Model file for the job. Use its own axes, mm. A direction names the side the tool comes from. Coordinates: 2 decimals unless noted, no trailing zeros. Write each loop counter-clockwise with the first axis right and the second up, starting at its lowest first coordinate (ties: lowest second). Pieces come first, ordered by that corner, then holes. Notation, with made-up numbers: M 2,8 L 27,8 A32 ccw 27,36 Z; hole C 40,11 d5. An arc over 180 degrees is marked long. Use CSV: the item, a comma, the result in double quotes. Start each with the question number.
from build123d import *

# Parameters (mm, degrees)
BOSS_EXTRUDE1_DEPTH = 10
SKETCH3_R           = 2.5
BOSS_EXTRUDE2_DEPTH = 10
FILLET1_R           = 2
RIB14_REACH         = 37
SKETCH5_WALL_W      = 93.213203436
SKETCH5_WALL_H      = 5


with BuildPart() as part:
    # Sketch2 → Boss-Extrude1 (new, symmetric)
    with BuildSketch(Plane(origin=(0, 0, 0), x_dir=(1, 0, 0), z_dir=(0, 1, 0))):
        Polygon((0, 15), (-15, 15), (-15, 20), (5, 20), (5, 0), (0, 0), align=None)
    extrude(amount=BOSS_EXTRUDE1_DEPTH, both=True)

    # Sketch3 → Boss-Extrude2 (add)
    with BuildSketch(Plane(origin=(0, 0, -20), x_dir=(-1, 0, 0), z_dir=(0, 0, -1))):
        with Locations((5, 0)):
            Circle(SKETCH3_R)
    extrude(amount=BOSS_EXTRUDE2_DEPTH)

    # Fillet1
    fillet1_edges = [part.edges().sort_by_distance(p)[0] for p in [
        (-2.5, 0, -30),
    ]]
    fillet(fillet1_edges, radius=FILLET1_R)

    # Sketch5 wall → Rib14 (add, up to next)
    with BuildSketch(Plane(origin=(-7.5, 0, -7.5), x_dir=(0.707106781187, 0, 0.707106781187), z_dir=(0.707106781187, 0, -0.707106781187)), mode=Mode.PRIVATE) as rib14_sk1:
        Rectangle(SKETCH5_WALL_W, SKETCH5_WALL_H)
    rib14_tool1 = extrude(rib14_sk1.sketch, amount=RIB14_REACH, mode=Mode.PRIVATE) - part.part
    add(rib14_tool1.solids().sort_by_distance((-7.5, 0, -7.5))[0])


solid = part.part
1) Wall check: L1, parallel to X at y = -4, z = -11; L2, parallel to Y at x = -2.25, z = -2.5; L3, parallel to Z at x = -6, y = 8. Give the ranges that are in metal, low to high. Write a range as [from, to].
2) Band-saw the part on C-C on z = -20.5. List the corners of the cut face in (x, y), then the cut area to 3 significant figures.
3) Tool access for faces 1 (the face through (-7, -6, -15)), 2 (the face through (-5, 0, -30)), 3 (the face through (-7, 6, -15)), 4 (the face through (-8, 0, -8)), 5 (the face through (-7.385, 0.751, -23.944)): list every direction of +Z, -Z, +X, -X, +Y, -Y with a clear straight run to the whole face (end or side of a thin tool).
4) Band-saw the part on A-A on z = -12. List the corners of the cut face in (x, y), then the cut area to 3 significant figures.
5) Band-saw the part on B-B on x = -1. List the corners of the cut face in (y, z).
6) Band-saw the part on D-D on x = 1. List the corners of the cut face in (y, z).
7) Drop flat-ended pins along their axis: P1, Ø8, axis at y = -4.5, z = -6, coming from the -X side; P2, Ø1, axis at x = -3, y = 5.5, coming from the +Z side; P3, Ø10, axis at x = -5, z = -23, coming from the -Y side; P4, Ø12, axis at x = -11, z = -4.5, coming from the +Y side. Give the stop position or say it passes through.
Findings below:
1,L1,"x = [0, 5]"
1,L2,"y = [-2.5, 2.5]"
1,L3,"z = [-20, -15]"
2,outline,"C -5,0 d5"
2,area,"19.6 mm2"
3,face 1,"+Z, -X, -Y"
3,face 2,"-Z, +X, -X, +Y, -Y"
3,face 3,"+Z, -X, +Y"
3,face 4,"+Z, -X, +Y, -Y"
3,face 5,"-Z"
4,outline,"M -12,-2.5 L 0,-2.5 L 0,-10 L 5,-10 L 5,10 L 0,10 L 0,2.5 L -12,2.5 Z"
4,area,"160 mm2"
5,outline,"M -10,-20 L 10,-20 L 10,-15 L 2.5,-15 L 2.5,-1 L -2.5,-1 L -2.5,-15 L -10,-15 Z"
6,outline,"M -10,-20 L 10,-20 L 10,0 L -10,0 Z"
7,P1,"stops at x = -9.46"
7,P2,"stops at z = -15"
7,P3,"stops at y = -10"
7,P4,"stops at y = 2.5"
